Verification items for this drawing (mm, ordinates from the low corner). A direction names the side the tool comes from. Round coordinates to 2 decimals unless told otherwise and drop trailing zeros. Write each loop counter-clockwise with the first axis right and the second up, starting at its lowest first coordinate (ties: lowest second). Pieces come first, ordered by that corner, then holes. Notation, with made-up numbers: (83.25, 13) -> (122.25, 13) arc R27 ccw to (122.25, 41) -> close; hole circle Ø5 at (42, 65.25). An arc over 180 degrees is marked (long way). Use one line per item in the form item = value. Start each with the question number.
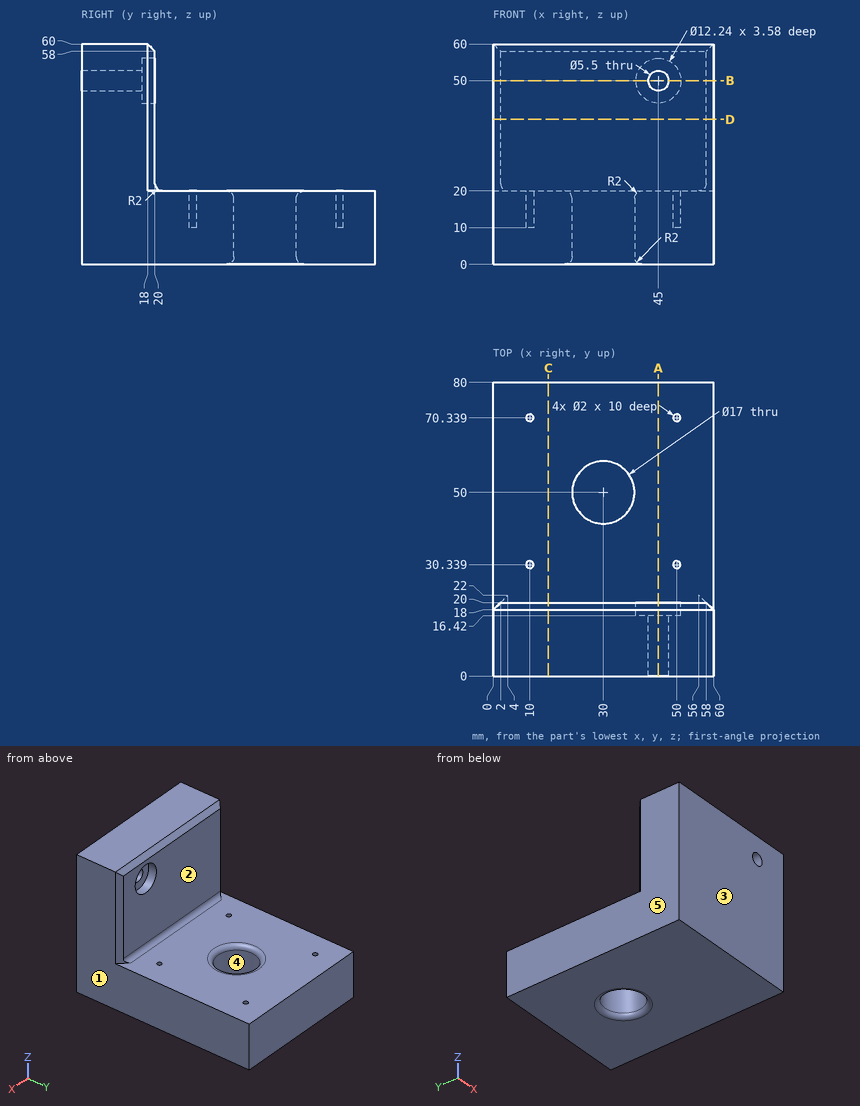
1. Sectioned sample at C-C (x = 15). Enter the section's corners in (y, z), and give its area (3 significant figures).
2. Sectioned sample at A-A (x = 45). Enter the section's corners in (y, z).
3. Mould release check, pull along X, two halves, no side actions. Record for the marked faces 3, 4 and 5: +X half, -X half, draft (parallel to the pull), parting line (faces both ways), or undercut.
4. Depth check by flat-ended pin: pin 1 (1 mm diameter, centred on x = 10, y = 30, fed in from +Z); pin 2 (2.5 mm diameter, centred on x = 10, y = 70.34, fed in from +Z); pin 3 (4 mm diameter, centred on x = 26, z = 36, fed in from +Y). Enter the tip coordinate at first touch or a pass-through.
5. Sectioned sample at B-B (z = 50). Enter the section's corners in (x, y).
6. Tool access check on the marked faces 1 and 2. Record the directions out of +Z, -Z, +X, -X, +Y, -Y that give a thin tool (end or side, any length) a straight path to the whole face; none if there is none.
7. Sectioned sample at D-D (z = 39.5). Enter the section's corners in (x, y), and give its area (3 significant figures).
8. Scan lines: probe 1 along Y at (x, z) = (50, 17.75); probe 2 along X at (y, z) = (3.5, 50); probe 3 along Z at (x, y) = (40, 53). Record each from-to range of solid material in increasing order.
Returned:
q1.outline = (0, 0) -> (80, 0) -> (80, 20) -> (22, 20) arc R2 cw to (20, 22) -> (20, 58) -> (18, 60) -> (0, 60) -> close
q1.area = 2,400 mm^2
q2.outline = (0, 0) -> (80, 0) -> (80, 20) -> (22, 20) arc R2 cw to (20, 22) -> (20, 43.88) -> (16.42, 43.88) -> (16.42, 47.25) -> (0, 47.25) -> close; (0, 52.75) -> (16.42, 52.75) -> (16.42, 56.12) -> (20, 56.12) -> (20, 58) -> (18, 60) -> (0, 60) -> close
q3.face_3 = draft
q3.face_4 = undercut
q3.face_5 = -X half
q4.pin_1 = 10
q4.pin_2 = 20
q4.pin_3 = 20
q5.outline = (0, 0) -> (42.25, 0) -> (42.25, 16.42) -> (38.88, 16.42) -> (38.88, 20) -> (2, 20) -> (0, 18) -> close; (47.75, 0) -> (60, 0) -> (60, 18) -> (58, 20) -> (51.12, 20) -> (51.12, 16.42) -> (47.75, 16.42) -> close
q6.face_1 = +Z, -Z, +X, +Y, -Y
q6.face_2 = +Z, +X, -X, +Y
q7.outline = (0, 0) -> (60, 0) -> (60, 18) -> (58, 20) -> (2, 20) -> (0, 18) -> close
q7.area = 1,200 mm^2
q8.probe_1 = 0 to 29.34, 31.34 to 69.34, 71.34 to 80
q8.probe_2 = 0 to 42.25, 47.75 to 60
q8.probe_3 = 0 to 20
